Check sheet for the modelled part. Datum: model origin and axes. Units: mm. Face numbers are marked on the shaded views. A direction names the side the tool comes from. Coordinates: 2 decimals unless noted, no trailing zeros. Write each loop counter-clockwise with the first axis right and the second up, starting at its lowest first coordinate (ties: lowest second). Pieces come first, ordered by that corner, then holes. Notation, with made-up numbers: (66, -2) - (76, -2) arc R32 ccw to (76, 33) - close; hole circle Ø11 at (36, 54). An arc over 180 degrees is marked (long way). Use one line per item in the form item = value. Start each with the question number.
1. Cross-section at B-B on y = 10.5. Record the boundary of the cut face in (x, z), then the cut area to 3 significant figures.
2. Tool access check on the marked faces 1 and 2. Record the directions out of +Z, -Z, +X, -X, +Y, -Y that give a thin tool (end or side, any length) a straight path to the whole face; none if there is none.
3. Go/stop test with flat-tipped pins: pin 1 Ø1.7 at (x, z) = (-4.5, 6.5) entering from -Y; pin 2 Ø8 at (y, z) = (10.5, 1.5) entering from +X; pin 3 Ø2 at (x, y) = (-13.5, 4.5) entering from -Z. Record where each tip stops, or that it passes through.
4. Draft check along X on the marked faces 3, 4 and 5. Enter one of: +X half, -X half, draft (parallel to the pull), parting line (faces both ways), or undercut.
5. Cross-section at A-A on y = 3.25. Record the boundary of the cut face in (x, z), then the cut area to 3 significant figures.
6. Scan lines: line 1 along X through (y, z) = (10, 0); line 2 along X through (y, z) = (4.9, -5.6); line 3 along X through (y, z) = (-0.6, -5.6). Record each from-to range of solid material in increasing order.
7. Cross-section at C-C on z = 5.6. Give the number of separate pieces and of enclosed holes in the cut face, then the cut area to 3 significant figures.
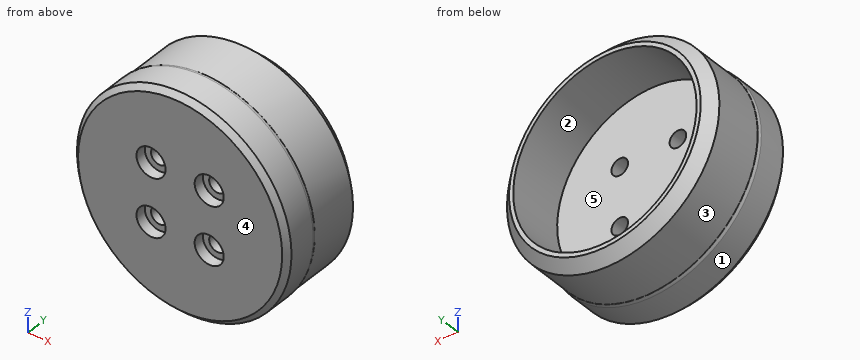
```python
from build123d import *

# Parameters (mm, degrees)
BOSS_EXTRUDE1_DEPTH      = 6.5
BOSS_EXTRUDE1_DEPTH_BACK = 1
SKETCH1_R                = 20.65
SKETCH2_R                = 20.45
SKETCH2_R_2              = 17.65
BOSS_EXTRUDE2_DEPTH      = 10.6
SKETCH4_R                = 1.6
CUT_EXTRUDE1_DEPTH       = 13.5
SKETCH8_R                = 2.8
CUT_EXTRUDE2_DEPTH       = 2
CHAMFER1_SIZE            = 1
CHAMFER3_SIZE            = 1
CHAMFER3_SIZE_2          = 0.577350269
FILLET1_R                = 1
CHAMFER4_SIZE            = 2


# Some blends are built 0.0001 mm under size
with BuildPart() as part:
    # Sketch1 → Boss-Extrude1 (new, two sides: drawn at the far end of the back side and taken through both)
    with BuildSketch(Plane(origin=(0, 0, 0), x_dir=(1, 0, 0), z_dir=(0, 1, 0)).offset(-BOSS_EXTRUDE1_DEPTH_BACK)):
        with Locations(Location((0, 0, 0), (0, 0, 270))):
            Circle(SKETCH1_R)
    extrude(amount=BOSS_EXTRUDE1_DEPTH + BOSS_EXTRUDE1_DEPTH_BACK)

    # Sketch2 → Boss-Extrude2 (add)
    with BuildSketch(Plane(origin=(0, 6.5, 0), x_dir=(1, 0, 0), z_dir=(0, 1, 0))):
        with Locations(Location((0, 0, 0), (0, 0, 270))):
            Circle(SKETCH2_R)
        with Locations(Location((0, 0, 0), (0, 0, 270))):
            Circle(SKETCH2_R_2, mode=Mode.SUBTRACT)
    extrude(amount=BOSS_EXTRUDE2_DEPTH)

    # Sketch4 → Cut-Extrude1 (cut)
    with BuildSketch(Plane.XZ.offset(1)):
        with Locations(Location((-5.6, 5.6, 0), (0, 0, 270))):
            Circle(SKETCH4_R)
        with Locations(Location((5.6, 5.6, 0), (0, 0, 270))):
            Circle(SKETCH4_R)
        with Locations(Location((5.6, -5.6, 0), (0, 0, 270))):
            Circle(SKETCH4_R)
        with Locations(Location((-5.6, -5.6, 0), (0, 0, 270))):
            Circle(SKETCH4_R)
    extrude(amount=-CUT_EXTRUDE1_DEPTH, mode=Mode.SUBTRACT)

    # Sketch8 → Cut-Extrude2 (cut)
    with BuildSketch(Plane.XZ.offset(1)):
        with Locations(Location((5.6, -5.6, 0), (0, 0, 270))):
            Circle(SKETCH8_R)
        with Locations(Location((-5.6, -5.6, 0), (0, 0, 270))):
            Circle(SKETCH8_R)
        with Locations(Location((-5.6, 5.6, 0), (0, 0, 270))):
            Circle(SKETCH8_R)
        with Locations(Location((5.6, 5.6, 0), (0, 0, 270))):
            Circle(SKETCH8_R)
    extrude(amount=-CUT_EXTRUDE2_DEPTH, mode=Mode.SUBTRACT)

    # Chamfer1
    chamfer1_edges = [part.edges().sort_by_distance(p)[0] for p in [
        (0, -1, -20.65),
    ]]
    chamfer(chamfer1_edges, length=CHAMFER1_SIZE - 0.0001)  # a hair under: the kernel refuses the full size

    # Chamfer3
    # the kernel refuses this chamfer: 1, 0.577350269 mm, written as the material it takes off along each edge
    with BuildSketch(Plane(origin=(0, 6.5, 0), x_dir=(0, 0, 1), z_dir=(-1, 0, 0))) as chamfer3_piece_1_section:
        Polygon((20.65, -CHAMFER3_SIZE), (20.65 - CHAMFER3_SIZE_2, 0), (20.65, 0), align=None)
    chamfer3_piece_1 = revolve(axis=Axis((0, 6.5, 0), (0, 1, 0)), mode=Mode.PRIVATE)
    chamfer3_piece_1 = chamfer3_piece_1 - Plane(origin=(0, 5.670486655, 0), x_dir=(0, 0, 1), z_dir=(0, -1, 0)) * Cylinder(20.45, 83, mode=Mode.PRIVATE)
    add(chamfer3_piece_1, mode=Mode.SUBTRACT)

    # Fillet1
    fillet1_edges = [part.edges().sort_by_distance(p)[0] for p in [
        (0, 5.5, -20.65),
    ]]
    fillet(fillet1_edges, radius=FILLET1_R)

    # Chamfer4
    chamfer4_edges = [part.edges().sort_by_distance(p)[0] for p in [
        (0, 17.1, -20.45),
    ]]
    chamfer(chamfer4_edges, length=CHAMFER4_SIZE)


solid = part.part
```
Final values:
q1.outline = circle Ø40.9 at (0, 0); hole circle Ø35.3 at (0, 0)
q1.area = 335 mm²
q2.face_1 = +Y, -Y
q2.face_2 = +Y
q3.pin_1 = 1
q3.pin_2 = 20.45
q3.pin_3 = -16.44
q4.face_3 = parting line
q4.face_4 = draft
q4.face_5 = undercut
q5.outline = circle Ø41.3 at (0, 0); hole circle Ø3.2 at (-5.6, -5.6); hole circle Ø3.2 at (-5.6, 5.6); hole circle Ø3.2 at (5.6, -5.6); hole circle Ø3.2 at (5.6, 5.6)
q5.area = 1,310 mm²
q6.line_1 = -20.45 to -17.65, 17.65 to 20.45
q6.line_2 = -19.88 to -7.2, -4 to 4, 7.2 to 19.88
q6.line_3 = -19.25 to -8.4, -2.8 to 2.8, 8.4 to 19.25
q7.separate_pieces = 3
q7.enclosed_holes = 0
q7.area = 297 mm²
